from build123d import *

# Parameters (mm, degrees)
SKETCH1_R                                           = 39
BOSS_EXTRUDE1_DEPTH                                 = 18.5
SKETCH2_R                                           = 37
CUT_EXTRUDE1_DEPTH                                  = 7.5
SKETCH3_R                                           = 26.5
CUT_EXTRUDE2_DEPTH                                  = 4
SKETCH4_R                                           = 17.5
BOSS_EXTRUDE2_DEPTH                                 = 5
SKETCH5_R                                           = 15
BOSS_EXTRUDE3_DEPTH                                 = 12
SKETCH6_R                                           = 6.25
SKETCH6_R_2                                         = 1.8
CUT_EXTRUDE3_DEPTH                                  = 25
CSK_FOR_M4_COUNTERSUNK_FLAT_HEAD_SCREW1_D           = 3.5
CSK_FOR_M4_COUNTERSUNK_FLAT_HEAD_SCREW1_CSINK_D     = 9.1
CSK_FOR_M4_COUNTERSUNK_FLAT_HEAD_SCREW1_CSINK_ANGLE = 90
SKETCH9_R                                           = 2.05
CUT_EXTRUDE4_DEPTH                                  = 12.0000001
CUT_EXTRUDE5_DEPTH                                  = 2.5
CIRPATTERN1_COUNT                                   = 6
SKETCH11_R                                          = 4
BOSS_EXTRUDE5_DEPTH                                 = 18.5


with BuildPart() as part:
    # Sketch1 → Boss-Extrude1 (new body)
    with BuildSketch(Plane(origin=(0, 0, 0), x_dir=(1, 0, 0), z_dir=(0, 1, 0))):
        Circle(SKETCH1_R)
    extrude(amount=BOSS_EXTRUDE1_DEPTH)

    # Sketch2 → Cut-Extrude1 (cut)
    with BuildSketch(Plane(origin=(0, 18.5, 0), x_dir=(1, 0, 0), z_dir=(0, 1, 0))):
        Circle(SKETCH2_R)
    extrude(amount=-CUT_EXTRUDE1_DEPTH, mode=Mode.SUBTRACT)

    # Sketch3 → Cut-Extrude2 (cut)
    with BuildSketch(Plane(origin=(0, 11, 0), x_dir=(1, 0, 0), z_dir=(0, 1, 0))):
        Circle(SKETCH3_R)
    extrude(amount=-CUT_EXTRUDE2_DEPTH, mode=Mode.SUBTRACT)

    # Sketch4 → Boss-Extrude2 (add)
    with BuildSketch(Plane(origin=(0, 7, 0), x_dir=(1, 0, 0), z_dir=(0, 1, 0))):
        Circle(SKETCH4_R)
    extrude(amount=BOSS_EXTRUDE2_DEPTH)

    # Sketch5 → Boss-Extrude3 (add)
    with BuildSketch(Plane(origin=(0, 12, 0), x_dir=(1, 0, 0), z_dir=(0, 1, 0))):
        Circle(SKETCH5_R)
    extrude(amount=BOSS_EXTRUDE3_DEPTH)

    # Sketch6 → Cut-Extrude3 (cut, through all)
    with BuildSketch(Plane(origin=(0, 24, 0), x_dir=(1, 0, 0), z_dir=(0, 1, 0))):
        Circle(SKETCH6_R)
        with Locations((0, 11)):
            Circle(SKETCH6_R_2)
        with Locations((11, 0)):
            Circle(SKETCH6_R_2)
        with Locations((0, -11)):
            Circle(SKETCH6_R_2)
        with Locations((-11, 0)):
            Circle(SKETCH6_R_2)
    extrude(amount=-CUT_EXTRUDE3_DEPTH, mode=Mode.SUBTRACT)

    # CSK for M4 Countersunk Flat Head Screw1 (through all)
    with Locations(Plane(origin=(0, 0, 11), x_dir=(0, 0, -1), z_dir=(0, -1, 0))):
        with Locations((0, 0), (11, 11), (22, 0), (11, -11)):
            CounterSinkHole(CSK_FOR_M4_COUNTERSUNK_FLAT_HEAD_SCREW1_D / 2, CSK_FOR_M4_COUNTERSUNK_FLAT_HEAD_SCREW1_CSINK_D / 2, counter_sink_angle=CSK_FOR_M4_COUNTERSUNK_FLAT_HEAD_SCREW1_CSINK_ANGLE)

    # Sketch9 → Cut-Extrude4 (cut, through all)
    with BuildSketch(Plane(origin=(0, 11, 0), x_dir=(1, 0, 0), z_dir=(0, 1, 0))):
        with Locations((0, 31.25)):
            Circle(SKETCH9_R)
        with Locations((27.063293868, 15.625)):
            Circle(SKETCH9_R)
        with Locations((27.063293868, -15.625)):
            Circle(SKETCH9_R)
        with Locations((0, -31.25)):
            Circle(SKETCH9_R)
        with Locations((-27.063293868, -15.625)):
            Circle(SKETCH9_R)
        with Locations((-27.063293868, 15.625)):
            Circle(SKETCH9_R)
    extrude(amount=-CUT_EXTRUDE4_DEPTH, mode=Mode.SUBTRACT)

    # Sketch10 → Cut-Extrude5 (cut)
    with BuildSketch(Plane(origin=(0, 11, 0), x_dir=(1, 0, 0), z_dir=(0, 1, 0))):
        Polygon((2.078460969, 34.85), (-2.078460969, 34.85), (-4.156921938, 31.25), (-2.078460969, 27.65), (2.078460969, 27.65), (4.156921938, 31.25), align=None)
    cut_extrude5 = extrude(amount=-CUT_EXTRUDE5_DEPTH, mode=Mode.SUBTRACT)

    # CirPattern1: Cut-Extrude5 ×6 about axis
    cirpattern1_axis = Axis((0, 0, 0), (0, 1, 0))
    for i in range(1, CIRPATTERN1_COUNT):
        add(cut_extrude5.rotate(cirpattern1_axis, i * 360 / CIRPATTERN1_COUNT), mode=Mode.SUBTRACT)

    # Sketch11 → Boss-Extrude5 (add, through all)
    with BuildSketch(Plane(origin=(0, 18.5, 0), x_dir=(1, 0, 0), z_dir=(0, 1, 0))):
        with Locations((-21.5, -37.239092363)):
            Circle(SKETCH11_R)
        with BuildLine():
            ThreePointArc((-17.5, -37.239092363), (-17.636296695, -38.274368543), (-18.035898385, -39.239092363))
            Line((-18.035898385, -39.239092363), (-15.933063126, -35.596874855))
            ThreePointArc((-15.933063126, -35.596874855), (-17.739935267, -34.731753436), (-19.499999848, -33.774990835))
            ThreePointArc((-19.499999848, -33.774990835), (-18.035898341, -35.239092439), (-17.5, -37.239092363))
        make_face()
        with BuildLine():
            Line((-22.861266356, -31.596874855), (-24.964101615, -35.239092363))
            ThreePointArc((-24.964101615, -35.239092363), (-22.535276096, -33.375389035), (-19.499999848, -33.774990835))
            ThreePointArc((-19.499999848, -33.774990835), (-21.208613012, -32.729111416), (-22.861266356, -31.596874855))
        make_face()
    extrude(amount=-BOSS_EXTRUDE5_DEPTH)


solid = part.part
Build history of the part. All positions in model axes, mm. A direction names the side the tool comes from. Round coordinates to 2 decimals unless told otherwise and drop trailing zeros. Loops run counter-clockwise (first coordinate to the right, second up) from the corner with the lowest first, then second, coordinate; pieces in that order, holes last. Notation, with made-up numbers: (-32, 12) -> (2, 12) arc R8 ccw to (2, 26) -> close; hole circle Ø9 at (26, 4.5). An arc over 180 degrees is marked (long way). Answer in a Markdown table with one row per item.
Item 1: Saw through at B-B (x = 11). Write the cut outline in (y, z), and give its area (3 significant figures).
Answers below:
| item | result |
|---|---|
| outline | (0, -37.42) -> (18.5, -37.42) -> (18.5, -35.33) -> (11, -35.33) -> (11, -24.11) -> (7, -24.11) -> (7, -13.61) -> (12, -13.61) -> (12, -10.2) -> (24, -10.2) -> (24, -1.8) -> (2.75, -1.8) -> (0, -4.55) -> close; (0, 4.55) -> (2.75, 1.8) -> (24, 1.8) -> (24, 10.2) -> (12, 10.2) -> (12, 13.61) -> (7, 13.61) -> (7, 24.11) -> (11, 24.11) -> (11, 35.33) -> (18.5, 35.33) -> (18.5, 37.42) -> (0, 37.42) -> close |
| area | 949 mm² |
Item 2: Saw through at A-A (y = 15.5). Write the cut outline in (x, z), and give its area (3 significant figures).
Answers below:
| item | result |
|---|---|
| outline | (-24.96, 35.24) -> (-22.86, 31.6) arc R39 ccw (long way) to (-15.93, 35.6) -> (-18.04, 39.24) arc R4 ccw to start; circle Ø30 at (0, 0); hole circle Ø74 at (0, 0); hole circle Ø3.6 at (-11, 0); hole circle Ø12.5 at (0, 0); hole circle Ø3.6 at (0, -11); hole circle Ø3.6 at (0, 11); hole circle Ø3.6 at (11, 0) |
| area | 1,080 mm² |
Item 3: Drill centre lines: L1, parallel to X at y = 9.55, z = 0; L2, parallel to X at y = 19.75, z = 0; L3, parallel to X at y = 17, z = -8. Where is each one in solid material? Low to high. Write a range as [from, to].
Answers below:
| item | result |
|---|---|
| L1 | x = [-39, -26.5], [-17.5, -12.8], [-9.2, -6.25], [6.25, 9.2], [12.8, 17.5], [26.5, 39] |
| L2 | x = [-15, -12.8], [-9.2, -6.25], [6.25, 9.2], [12.8, 15] |
| L3 | x = [-38.17, -36.12], [-12.69, 12.69], [36.12, 38.17] |
Item 4: Mould opens along Z. For faces 4 (the flat face through (-29.4, 8.5, 14.9)), 5 (the flat face through (-16.999, 9.38, 37.443)) say: +Z half, -Z half, draft (parallel to the pull), parting line (faces both ways), or undercut.
Answers below:
| item | result |
|---|---|
| face 4 | undercut |
| face 5 | +Z half |
Item 5: Saw through at D-D (z = 11). Write the cut outline in (x, y), and give its area (3 significant figures).
Answers below:
| item | result |
|---|---|
| outline | (-37.42, 0) -> (-4.55, 0) -> (-1.8, 2.75) -> (-1.8, 24) -> (-10.2, 24) -> (-10.2, 12) -> (-13.61, 12) -> (-13.61, 7) -> (-24.11, 7) -> (-24.11, 11) -> (-35.33, 11) -> (-35.33, 18.5) -> (-37.42, 18.5) -> close; (1.8, 2.75) -> (4.55, 0) -> (37.42, 0) -> (37.42, 18.5) -> (35.33, 18.5) -> (35.33, 11) -> (24.11, 11) -> (24.11, 7) -> (13.61, 7) -> (13.61, 12) -> (10.2, 12) -> (10.2, 24) -> (1.8, 24) -> close |
| area | 949 mm² |
Item 6: Saw through at C-C (y = 21.25). Write the cut outline in (x, z).
Answers below:
| item | result |
|---|---|
| outline | circle Ø30 at (0, 0); hole circle Ø3.6 at (-11, 0); hole circle Ø12.5 at (0, 0); hole circle Ø3.6 at (0, -11); hole circle Ø3.6 at (0, 11); hole circle Ø3.6 at (11, 0) |
Item 7: Pin check, flat tips, straight feed: pin 1 (5.5 mm diameter, centred on x = 0, z = 31.25, fed in from +Y); pin 2 (3 mm diameter, centred on x = 20.5, z = -13, fed in from -Y); pin 3 (5 mm diameter, centred on y = 2.5, z = -30, fed in from -X); pin 4 (1 mm diameter, centred on x = -3.5, y = 21.5, fed in from -Z). Stop position of each tip, or through.
Answers below:
| item | result |
|---|---|
| pin 1 | stops at y = 8.5 |
| pin 2 | stops at y = 0 |
| pin 3 | stops at x = -27.65 |
| pin 4 | stops at z = -14.7 |
Item 8: Which spindle directions (+Z, -Z, +X, -X, +Y, -Y) get a long thin tool onto all of the face, cutting with end or side? Do faces 1 (the cylindrical face through (25.015, 4.31, -15.715)), 2 (the flat face through (-23.9, 9.8, 13.9)), 3 (the flat face through (-23.9, 9.4, 33.4)). Say none if no direction does.
Answers below:
| item | result |
|---|---|
| face 1 | +Y, -Y |
| face 2 | +Y |
| face 3 | -X, +Y, -Y |
